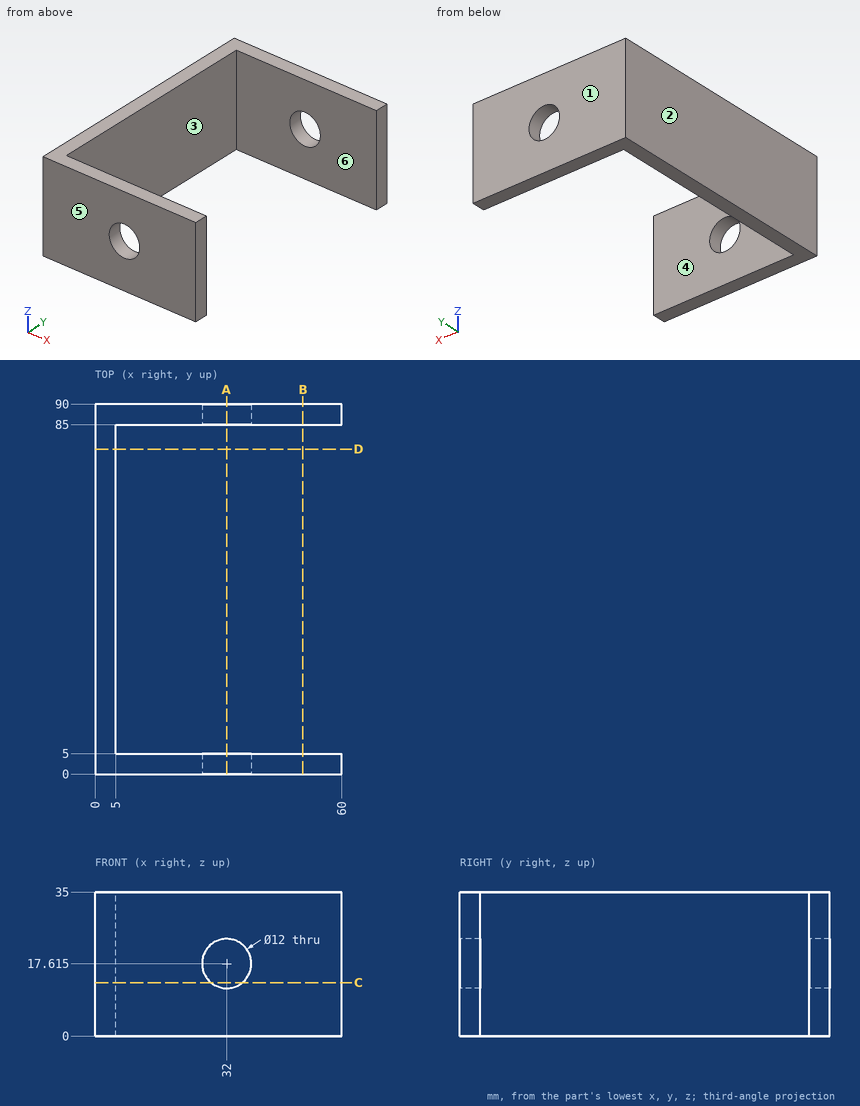
Could you check a few things on this drawing? It's one solid part, dimensions in mm from its lowest x, y, z. A direction names the side the tool comes from. Give positions to 0.01 mm unless a question says otherwise; leave off trailing zeros. Write each loop counter-clockwise with the first axis right and the second up, starting at its lowest first coordinate (ties: lowest second). Pieces come first, ordered by that corner, then holes. Notation, with made-up numbers: (-34.5, -37) -> (-12.5, -37) arc R27 cw to (-12.5, -7) -> close; hole circle Ø9 at (65.5, 30). An arc over 180 degrees is marked (long way). Write item = value, one per line.
(1) Suppose I cut it at D-D on y = 79. Write out the boundary of the cut face in (x, z), then the cut area to 3 significant figures.
Worked out:
outline = (0, 0) -> (5, 0) -> (5, 35) -> (0, 35) -> close
area = 175 mm^2
(2) Suppose I cut it at A-A on x = 32. Write out the boundary of the cut face in (y, z) (1 decimal).
Worked out:
outline = (0, 0) -> (5, 0) -> (5, 11.6) -> (0, 11.6) -> close; (0, 23.6) -> (5, 23.6) -> (5, 35) -> (0, 35) -> close; (85, 0) -> (90, 0) -> (90, 11.6) -> (85, 11.6) -> close; (85, 23.6) -> (90, 23.6) -> (90, 35) -> (85, 35) -> close
(3) Thinking about a two-plate mould opening in Y: for the marked faces 1, 2, 3 and 4, which applies, released by +Y, released by -Y, zero draft, split by the parting line, or undercut?
Worked out:
face_1 = released by +Y
face_2 = zero draft
face_3 = undercut
face_4 = undercut
(4) I'm going to push flat-ended pins straight in: P1, Ø4, axis at y = 39, z = 21, coming from the +X side; P2, Ø17.5, axis at x = 44, z = 20.5, coming from the -Y side; P3, Ø9.5, axis at x = 32, z = 17.61, coming from the +Y side. Where does each tip first touch, or does it pass through?
Worked out:
P1 = 5
P2 = 0
P3 = through
(5) Suppose I cut it at B-B on x = 50.5. Write out the boundary of the cut face in (y, z), then the cut area to 3 significant figures.
Worked out:
outline = (0, 0) -> (5, 0) -> (5, 35) -> (0, 35) -> close; (85, 0) -> (90, 0) -> (90, 35) -> (85, 35) -> close
area = 350 mm^2
(6) For the marked faces 5 and 6, which set-ups out of +Z, -Z, +X, -X, +Y, -Y let a thin tool reach every point of the face, with its end or its side?
Worked out:
face_5 = +Z, -Z, +X, -X, -Y
face_6 = +Z, -Z, +X
(7) I need wall thicknesses on probe 1 along Y at (x, z) = (26.5, 4); probe 2 along Z at (x, y) = (32, 87) (1 decimal); probe 3 along X at (y, z) = (7, 26). Which ranges of each line are inside material? Lowest first, please. Write a range as from..to.
Worked out:
probe_1 = 0..5, 85..90
probe_2 = 0..11.6, 23.6..35
probe_3 = 0..5
(8) Suppose I cut it at C-C on z = 13. Write out the boundary of the cut face in (x, y) (1 decimal).
Worked out:
outline = (0, 0) -> (28.2, 0) -> (28.2, 5) -> (5, 5) -> (5, 85) -> (28.2, 85) -> (28.2, 90) -> (0, 90) -> close; (35.8, 0) -> (60, 0) -> (60, 5) -> (35.8, 5) -> close; (35.8, 85) -> (60, 85) -> (60, 90) -> (35.8, 90) -> close
